from build123d import *

# Parameters (mm, degrees)
SALIENTE_EXTRUIR1_DEPTH = 9.525
SALIENTE_EXTRUIR2_DEPTH = 9.525


with BuildPart() as part:
    # Croquis1 → Saliente-Extruir1 (new body)
    with BuildSketch(Plane(origin=(0, 0, 0), x_dir=(1, 0, 0), z_dir=(0, 1, 0))):
        Polygon((0, 0), (0, 76.2), (76.2, 0), align=None)
    extrude(amount=SALIENTE_EXTRUIR1_DEPTH)

    # Croquis2 → Saliente-Extruir2 (add)
    with BuildSketch(Plane(origin=(0, 9.525, 0), x_dir=(1, 0, 0), z_dir=(0, 1, 0))):
        Polygon((76.2, 0), (76.2, 9.525), (9.525, 76.2), (0, 76.2), align=None)
    extrude(amount=-SALIENTE_EXTRUIR2_DEPTH)


solid = part.part
The model under review builds one solid part; all positions refer to its coordinate system, in mm. Round coordinates to 2 decimals unless told otherwise and drop trailing zeros. Order: outer loops, then holes, each group sorted by start corner. A loop starts at its lowest first (then second) coordinate and runs counter-clockwise, first axis right, second up. Notation, with made-up numbers: (-18.5, 6) -> (-7.5, 6) arc R21 cw to (-7.5, 41) -> close; hole circle Ø8 at (47, -35.75). An arc over 180 degrees is marked (long way). Write item = value, one per line. Start each with the question number.
Item 1: Consider section A-A on y = 4.5. Write out the cut boundary in (x, z) (3 decimals).
Item 2: Consider section C-C on x = 30. Write out the cut boundary in (y, z) (3 decimals), plus the area to 3 significant figures.
Item 3: Clearance check with flat-ended pins moving along their axes: pin 1 Ø1 at (y, z) = (5.5, -26.5) entering from +X (3 decimals); pin 2 Ø2 at (x, y) = (13, 5.5) entering from -Z (3 decimals); pin 3 Ø4 at (y, z) = (4.5, -56.5) entering from +X (3 decimals). State where each tip first meets the part, or that it passes through.
Item 4: For line 1 along X through (y, z) = (6.5, -67) (3 decimals); line 2 along Z through (x, y) = (63.5, 5.25) (3 decimals); line 3 along X through (y, z) = (8.75, -63) (3 decimals), list the stretches that pass through material, from the lowest coordinate up.
Item 5: Consider section B-B on z = -19.5. Write out the cut boundary in (x, y) (3 decimals).
Conclusion:
q1.outline = (0, -76.2) -> (9.525, -76.2) -> (76.2, -9.525) -> (76.2, 0) -> (0, 0) -> close
q2.outline = (0, -55.725) -> (9.525, -55.725) -> (9.525, 0) -> (0, 0) -> close
q2.area = 531 mm2
q3.pin_1 = 59.725
q3.pin_2 = -73.725
q3.pin_3 = 31.225
q4.line_1 = 0 to 18.725
q4.line_2 = -22.225 to 0
q4.line_3 = 0 to 22.725
q5.outline = (0, 0) -> (66.225, 0) -> (66.225, 9.525) -> (0, 9.525) -> close
